Verification items for the finished model (mm, model axes). A direction names the side the tool comes from. Give positions to 0.01 mm unless a question says otherwise; leave off trailing zeros. Loops run counter-clockwise (first coordinate to the right, second up) from the corner with the lowest first, then second, coordinate; pieces in that order, holes last. Notation, with made-up numbers: (50, 68) - (55, 68) arc R25 ccw to (55, 88) - close; hole circle Ø7 at (-27, -11). An arc over 180 degrees is marked (long way). Put each result on its own line as item: value. Start each with the question number.
```python
from build123d import *

# Parameters (mm, degrees)
EXTRUDE_1_DEPTH     = 200
SKETCH_2_R          = 1.5
SKETCH_2_R_2        = 0.95
CUT_EXTRUDE_1_DEPTH = 5
FILLET_1_R          = 2


with BuildPart() as part:
    # Эскиз1 → Вытянуть1 (new body)
    with BuildSketch(Plane.XY):
        with BuildLine():
            Line((0, 0), (1.5, 0))
            Line((1.5, 0), (1.5, 7))
            ThreePointArc((1.5, 7), (1.939339828, 8.060660172), (3, 8.5))
            Line((3, 8.5), (10, 8.5))
            Line((10, 8.5), (10, 10))
            Line((10, 10), (3, 10))
            ThreePointArc((3, 10), (0.878679656, 9.121320344), (0, 7))
            Line((0, 7), (0, 0))
        make_face()
    extrude(amount=EXTRUDE_1_DEPTH)

    # Эскиз2 → Вырез-Вытянуть1 (cut)
    with BuildSketch(Plane(origin=(0, 10, 0), x_dir=(-1, 0, 0), z_dir=(0, 1, 0))):
        with Locations(Location((-4, 196, 0), (0, 0, 48.189685104))):
            Circle(SKETCH_2_R)
        with Locations(Location((-4, 4, 0), (0, 0, 48.189685104))):
            Circle(SKETCH_2_R)
        with Locations((-4, -88)):
            Circle(SKETCH_2_R_2)
    extrude(amount=-CUT_EXTRUDE_1_DEPTH, mode=Mode.SUBTRACT)

    # Скругление1
    fillet_1_edges = [part.edges().sort_by_distance(p)[0] for p in [
        (10, 9.25, 200),
        (0.75, 0, 200),
        (10, 9.25, 0),
        (0.75, 0, 0),
    ]]
    fillet(fillet_1_edges, radius=FILLET_1_R)


solid = part.part
```
1) Set-up check for faces 1 (the face through (1.5, 3, 99)), 2 (the face through (7, 10, 99)): record each of +Z, -Z, +X, -X, +Y, -Y from which the full face is reachable in a straight line by a thin tool's end or side.
2) Section check A-A, the plane z = 40. Enter the section's corners in (x, y), plus the area to 3 significant figures.
3) Scan lines: line 1 along Z through (x, y) = (4, 8.8); line 2 along X through (y, z) = (6, 71); line 3 along Y through (x, z) = (4, 155). Record each from-to range of solid material in increasing order. Write a range as from..to.
4) Section check B-B, the plane y = 3.75. Enter the section's corners in (x, z).
5) Depth check by flat-ended pin: P1, Ø4, axis at x = 2.5, z = 158.5, coming from the -Y side; P2, Ø2.5, axis at x = 4, z = 4, coming from the +Y side; P3, Ø5.5, axis at x = 8, z = 51.5, coming from the -Y side; P4, Ø1.5, axis at x = 2.5, z = 163, coming from the -Y side. Enter the tip coordinate at first touch or a pass-through.
Results are:
1. face 1: +Z, -Z, +X, -Y
1. face 2: +Z, -Z, +X, -X, +Y
2. outline: (0, 0) - (1.5, 0) - (1.5, 7) arc R1.5 cw to (3, 8.5) - (10, 8.5) - (10, 10) - (3, 10) arc R3 ccw to (0, 7) - close
2. area: 26.3 mm2
3. line 1: z = 0..2.5, 5.5..194.5, 197.5..200
3. line 2: x = 0..1.5
3. line 3: y = 8.5..10
4. outline: (0, 0) - (1.5, 0) - (1.5, 200) - (0, 200) - close
5. P1: stops at y = 0
5. P2: passes through
5. P3: stops at y = 8.5
5. P4: stops at y = 7.83
